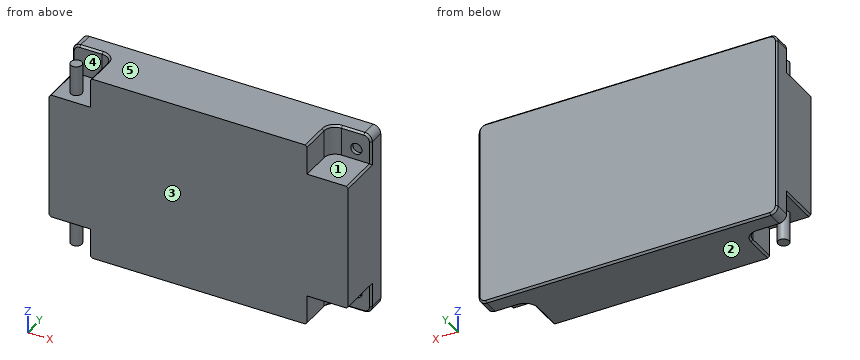
```python
from build123d import *

# Parameters (mm, degrees)
SKETCH1_W            = 800
SKETCH1_H            = 500
BOSS_EXTRUDE1_DEPTH  = 160
SKETCH3_W            = 110
SKETCH3_H            = 110
CUT_EXTRUDE1_DEPTH   = 80
FILLET1_R            = 30
FILLET1_OF_MIRROR1_R = 30
MIRROR2_START        = -250
MIRROR2_DEPTH        = 80
SHELL2_START         = -240
SHELL2_DEPTH         = 480
SHELL2_START_2       = -160
SHELL2_2_DEPTH       = 320
FILLET2_R            = 20
CHAMFER1_SIZE        = 5
CHAMFER2_SIZE        = 5
SKETCH7_R            = 15
BOSS_EXTRUDE2_DEPTH  = 80
SKETCH8_R            = 15
CUT_EXTRUDE2_DEPTH   = 20


# Read off the part's stored shape, not the designer's step: Mirror2, Shell2
with BuildPart() as part:
    # Sketch1 → Boss-Extrude1 (new body)
    with BuildSketch(Plane(origin=(0, 0, 0), x_dir=(1, 0, 0), z_dir=(0, 1, 0))):
        Rectangle(SKETCH1_W, SKETCH1_H)
    extrude(amount=BOSS_EXTRUDE1_DEPTH)

    # Sketch3 → Cut-Extrude1 (cut)
    with BuildSketch(Plane.XY.offset(250)):
        with Locations((-345, 55)):
            Rectangle(SKETCH3_W, SKETCH3_H)
    cut_extrude1 = extrude(amount=-CUT_EXTRUDE1_DEPTH, mode=Mode.SUBTRACT)

    # Fillet1
    fillet1_edges = [part.edges().sort_by_distance(p)[0] for p in [
        (-290, 110, 210),
    ]]
    fillet(fillet1_edges, radius=FILLET1_R)

    # Mirror1: Cut-Extrude1 across plane
    add(cut_extrude1.mirror(Plane(origin=(0, 0, 0), x_dir=(0, 0, 1), z_dir=(1, 0, 0))), mode=Mode.SUBTRACT)

    # Fillet1 of Mirror1
    fillet1_of_mirror1_edges = [part.edges().sort_by_distance(p)[0] for p in [
        (290, 110, 210),
    ]]
    fillet(fillet1_of_mirror1_edges, radius=FILLET1_OF_MIRROR1_R)

    # Mirror2 outline → Mirror2 (cut)
    with BuildSketch(Plane.XY.offset(MIRROR2_START)):
        with BuildLine():
            Line((400, 0), (400, 110))
            Line((400, 110), (320, 110))
            ThreePointArc((320, 110), (298.786796564, 101.213203436), (290, 80))
            Line((290, 80), (290, 0))
            Line((290, 0), (400, 0))
        make_face()
        with BuildLine():
            Line((-400, 0), (-290, 0))
            Line((-290, 0), (-290, 80))
            ThreePointArc((-290, 80), (-298.786796564, 101.213203436), (-320, 110))
            Line((-320, 110), (-400, 110))
            Line((-400, 110), (-400, 0))
        make_face()
    extrude(amount=MIRROR2_DEPTH, mode=Mode.SUBTRACT)

    # Shell2 outline → Shell2 (cut)
    with BuildSketch(Plane.XY.offset(SHELL2_START)):
        with BuildLine():
            Line((-280, 10), (280, 10))
            Line((280, 10), (280, 80))
            ThreePointArc((280, 80), (291.715728753, 108.284271247), (320, 120))
            Line((320, 120), (390, 120))
            Line((390, 120), (390, 150))
            Line((390, 150), (-390, 150))
            Line((-390, 150), (-390, 120))
            Line((-390, 120), (-320, 120))
            ThreePointArc((-320, 120), (-291.715728753, 108.284271247), (-280, 80))
            Line((-280, 80), (-280, 10))
        make_face()
    extrude(amount=SHELL2_DEPTH, mode=Mode.SUBTRACT)

    # Shell2 2 outline → Shell2 2 (cut)
    with BuildSketch(Plane.XY.offset(SHELL2_START_2)):
        with BuildLine():
            Line((280, 10), (390, 10))
            Line((390, 10), (390, 120))
            Line((390, 120), (320, 120))
            ThreePointArc((320, 120), (291.715728753, 108.284271247), (280, 80))
            Line((280, 80), (280, 10))
        make_face()
        with BuildLine():
            Line((-390, 10), (-280, 10))
            Line((-280, 10), (-280, 80))
            ThreePointArc((-280, 80), (-291.715728753, 108.284271247), (-320, 120))
            Line((-320, 120), (-390, 120))
            Line((-390, 120), (-390, 10))
        make_face()
    extrude(amount=SHELL2_2_DEPTH, mode=Mode.SUBTRACT)

    # Fillet2
    fillet2_edges = [part.edges().sort_by_distance(p)[0] for p in [
        (400, 135, 250),
        (-400, 135, 250),
        (-400, 135, -250),
        (400, 135, -250),
    ]]
    fillet(fillet2_edges, radius=FILLET2_R)

    # Chamfer1
    chamfer1_edges = [part.edges().sort_by_distance(p)[0] for p in [
        (-394.142135624, 110, 244.142135624),
        (394.142135624, 110, 244.142135624),
        (394.142135624, 110, -244.142135624),
        (-394.142135624, 110, -244.142135624),
        (-400, 55, 170),
        (-400, 110, 200),
        (-290, 40, 250),
        (-350, 110, 250),
        (-298.786796564, 101.213203436, 250),
        (400, 110, 200),
        (290, 40, 250),
        (400, 55, 170),
        (350, 110, 250),
        (298.786796564, 101.213203436, 250),
        (400, 55, -170),
        (400, 110, -200),
        (290, 40, -250),
        (350, 110, -250),
        (298.786796564, 101.213203436, -250),
        (-400, 110, -200),
        (-290, 40, -250),
        (-400, 55, -170),
        (-350, 110, -250),
        (-298.786796564, 101.213203436, -250),
    ]]
    chamfer(chamfer1_edges, length=CHAMFER1_SIZE)

    # Chamfer2
    chamfer2_edges = [part.edges().sort_by_distance(p)[0] for p in [
        (0, 160, 250),
        (-400, 160, 0),
        (400, 160, 0),
        (0, 160, -250),
        (-394.142135624, 160, -244.142135624),
        (394.142135624, 160, -244.142135624),
        (394.142135624, 160, 244.142135624),
        (-394.142135624, 160, 244.142135624),
    ]]
    chamfer(chamfer2_edges, length=CHAMFER2_SIZE)

    # Sketch7 → Boss-Extrude2 (add)
    with BuildSketch(Plane.XY.offset(170)):
        with Locations(Location((-350, 40, 0), (0, 0, 180))):
            Circle(SKETCH7_R)
    boss_extrude2 = extrude(amount=BOSS_EXTRUDE2_DEPTH)

    # Mirror3: Boss-Extrude2 across plane
    add(boss_extrude2.mirror(Plane.XY))

    # Sketch8 → Cut-Extrude2 (cut)
    with BuildSketch(Plane.XZ.offset(-110)):
        with Locations(Location((360, 200, 0), (0, 0, 270))):
            Circle(SKETCH8_R)
    cut_extrude2 = extrude(amount=-CUT_EXTRUDE2_DEPTH, mode=Mode.SUBTRACT)

    # Mirror4: Cut-Extrude2 across plane
    add(cut_extrude2.mirror(Plane.XY), mode=Mode.SUBTRACT)


solid = part.part
```
Design review of the part built by this model. Coordinates are the model's own, in mm. Face numbers are marked on the shaded views. A direction names the side the tool comes from. Coordinates: 2 decimals unless noted, no trailing zeros. Write each loop counter-clockwise with the first axis right and the second up, starting at its lowest first coordinate (ties: lowest second). Pieces come first, ordered by that corner, then holes.
1) To check wall thickness, follow L1, parallel to Y at x = 246.5, z = 57; L2, parallel to Z at x = 251.5, y = 78.5; L3, parallel to Z at x = 335, y = 59. State the ranges of each line that lie inside material, in increasing order.
2) Insertion check: pin 1 (6 mm diameter, centred on x = -310.5, y = 108.5, fed in from -Z); pin 2 (4 mm diameter, centred on y = 64, z = 189, fed in from +X); pin 3 (22.5 mm diameter, centred on x = -349, z = -210, fed in from -Y). Each pin has a flat end and moves straight along its axis. Give the tip position at first contact, or say it passes through.
3) Add section C-C (x = -225). Write out the cut boundary in (y, z).
4) Add section A-A (x = 360). Write out the cut boundary in (y, z), plus the area to 4 significant figures.
5) Add section B-B (z = 66). Write out the cut boundary in (x, y), plus the area to 3 significant figures.
6) Mouldability with a two-part tool opening along Y and no side actions: class the marked faces 3, 4 and 5 as +Y half, -Y half, draft (parallel to the pull), parting line (faces both ways), or undercut.
7) Machinability: for the marked faces 1 and 2, which of the approach directions +Z, -Z, +X, -X, +Y, -Y give a long, thin tool a straight path to every point of the face, cutting with its end or side? Answer none if there is none.
Check result:
1. L1: y = 0 to 10, 150 to 160
1. L2: z = -250 to -240, 240 to 250
1. L3: z = -170 to -160, 160 to 170
2. pin 1: stops at z = -248.04
2. pin 2: stops at x = 290
2. pin 3: stops at y = 25
3. outline: (0, -250) - (155, -250) - (160, -245) - (160, 245) - (155, 250) - (0, 250) - close; hole (10, -240) - (150, -240) - (150, 240) - (10, 240) - close
4. outline: (0, -170) - (110, -170) - (110, -185) - (120, -185) - (120, -160) - (10, -160) - (10, 160) - (120, 160) - (120, 185) - (110, 185) - (110, 170) - (0, 170) - close; (110, -245) - (115, -250) - (155, -250) - (160, -245) - (160, 245) - (155, 250) - (115, 250) - (110, 245) - (110, 215) - (120, 215) - (120, 240) - (150, 240) - (150, -240) - (120, -240) - (120, -215) - (110, -215) - close
4. area: 12,150 mm2
5. outline: (-400, 0) - (400, 0) - (400, 155) - (395, 160) - (-395, 160) - (-400, 155) - close; hole (-390, 10) - (390, 10) - (390, 150) - (-390, 150) - close
5. area: 18,800 mm2
6. face 3: -Y half
6. face 4: undercut
6. face 5: draft
7. face 1: +Z, +X, -Y
7. face 2: -Z, +X, -X, +Y, -Y
